Work out the finished part from the listing and answer in its coordinate system (mm). Coordinates: 2 decimals unless noted, no trailing zeros. Order: outer loops, then holes, each group sorted by start corner. A loop starts at its lowest first (then second) coordinate and runs counter-clockwise, first axis right, second up.
1. The part is cut by section C-C, the plane z = 84. Give the vertices of the cut face in (x, y) (3 decimals).
2. The part is cut by section B-B, the plane y = 1.2. Count the separate pieces of the cut face and the enclosed holes in it, then the cut area to 3 significant figures.
3. Find the intervals of material crossed by probe 1 along Z at (x, y) = (-55.5, 1.05); probe 2 along X at (y, z) = (1.2, 25.4); probe 3 along X at (y, z) = (0.7, -76.5), in increasing order.
4. The part is cut by section A-A, the plane z = -37. Give the vertices of the cut face in (x, y) (3 decimals).
5. Flat-ended cylindrical pins translate along their axes: pin 1 Ø8 at (x, z) = (-24.5, -38.5) entering from -Y; pin 2 Ø2 at (x, z) = (-120.45, 3.31) entering from -Y. Find the tip coordinate at first contact, or state that the pin passes through.
```python
from build123d import *

# Parameters (mm, degrees)
BOSS_EXTRUDE1_DEPTH         = 3.175
SKETCH3_W                   = 53.34
SKETCH3_H                   = 177.8
CUT_EXTRUDE1_DEPTH          = 3.175
F_27_0_144_DIAMETER_HOLE2_D = 3.6576
F_27_0_144_DIAMETER_HOLE3_D = 3.6576
SKETCH12_W                  = 127
SKETCH12_H                  = 254
CUT_EXTRUDE2_DEPTH          = 25.4


with BuildPart() as part:
    # Sketch2 → Boss-Extrude1 (new body)
    with BuildSketch(Plane(origin=(0, 0, 0), x_dir=(1, 0, 0), z_dir=(0, 1, 0))):
        with BuildLine():
            Line((-106.934, -102.87), (106.934, -102.87))
            ThreePointArc((106.934, -102.87), (122.020830283, -96.620830283), (128.27, -81.534))
            Line((128.27, -81.534), (128.27, 81.534))
            ThreePointArc((128.27, 81.534), (122.020830283, 96.620830283), (106.934, 102.87))
            Line((106.934, 102.87), (-106.934, 102.87))
            ThreePointArc((-106.934, 102.87), (-122.020830283, 96.620830283), (-128.27, 81.534))
            Line((-128.27, 81.534), (-128.27, -81.534))
            ThreePointArc((-128.27, -81.534), (-122.020830283, -96.620830283), (-106.934, -102.87))
        make_face()
    extrude(amount=BOSS_EXTRUDE1_DEPTH)

    # Sketch3 → Cut-Extrude1 (cut)
    with BuildSketch(Plane(origin=(0, 0, 0), x_dir=(1, 0, 0), z_dir=(0, 1, 0))):
        with Locations((-63.5, 0)):
            Rectangle(SKETCH3_W, SKETCH3_H)
    extrude(amount=CUT_EXTRUDE1_DEPTH, mode=Mode.SUBTRACT)

    # #27 (0.144) Diameter Hole2 (through all)
    with Locations(Plane(origin=(0, 3.175, 0), x_dir=(1, 0, 0), z_dir=(0, 1, 0))):
        with Locations((-24.13, -25.4), (-24.13, 88.9), (-102.87, 88.9), (-102.87, -25.4), (-102.87, -88.9), (-24.13, -88.9)):
            Hole(F_27_0_144_DIAMETER_HOLE2_D / 2)

    # #27 (0.144) Diameter Hole3 (through all)
    with Locations(Plane(origin=(0, 3.175, 0), x_dir=(1, 0, 0), z_dir=(0, 1, 0))):
        with Locations((-42.1132, 95.7453), (42.1132, 95.7453), (117.221, 92.2909), (117.6274, -92.5195), (49.403, -95.3643), (120.4468, -3.3147), (-49.403, -95.3643), (-117.6274, -92.5195), (-120.4468, -3.3147), (-117.221, 92.2909)):
            Hole(F_27_0_144_DIAMETER_HOLE3_D / 2)

    # Sketch12 → Cut-Extrude2 (cut)
    with BuildSketch(Plane(origin=(0, 3.175, 0), x_dir=(1, 0, 0), z_dir=(0, 1, 0))):
        with Locations((123.5456, 0)):
            Rectangle(SKETCH12_W, SKETCH12_H)
    extrude(amount=-CUT_EXTRUDE2_DEPTH, mode=Mode.SUBTRACT)


solid = part.part
```
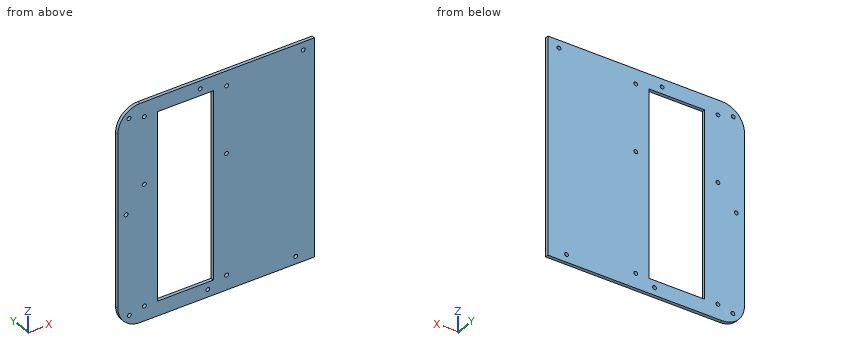
Geometry says:
1. outline: (-128.127, 0) - (-90.17, 0) - (-90.17, 3.175) - (-128.127, 3.175) - close; (-36.83, 0) - (60.046, 0) - (60.046, 3.175) - (-36.83, 3.175) - close
2. separate pieces: 1
2. enclosed holes: 14
2. area: 28,900 mm2
3. probe 1: z = -102.87 to -88.9, 88.9 to 102.87
3. probe 2: x = -128.27 to -104.7, -101.04 to -90.17, -36.83 to -25.96, -22.3 to 60.05
3. probe 3: x = -128.27 to -90.17, -36.83 to 60.05
4. outline: (-128.27, 0) - (-90.17, 0) - (-90.17, 3.175) - (-128.27, 3.175) - close; (-36.83, 0) - (60.046, 0) - (60.046, 3.175) - (-36.83, 3.175) - close
5. pin 1: stops at y = 0
5. pin 2: passes through
